```python
from build123d import *

# Parameters (mm, degrees)
F0_W      = 270
F0_H      = 280
F1_DEPTH  = 3
F2_R      = 2.25
F3_DEPTH  = 3.001
F4_R      = 2.25
F5_DEPTH  = 3.001
F7_DEPTH  = 3.001
F8_DEPTH  = 100
F9_R      = 2.25
F10_DEPTH = 3.001
F11_W     = 18
F11_H     = 20
F12_DEPTH = 3.001
F13_R     = 15


with BuildPart() as f1:
    # F0 (on Top) → F1 (new body)
    with BuildSketch(Plane.XY):
        Rectangle(F0_W, F0_H)
    extrude(amount=F1_DEPTH)

    # F2 (on face) → F3 (cut, through all)
    with BuildSketch(Plane.XY.offset(3)):
        with Locations((-16, -130)):
            Circle(F2_R)
        with Locations((-16, -90)):
            Circle(F2_R)
        with Locations((16, -130)):
            Circle(F2_R)
        with Locations((16, -90)):
            Circle(F2_R)
        with Locations((16, 118)):
            Circle(F2_R)
        with Locations((16, 78)):
            Circle(F2_R)
        with Locations((-16, 78)):
            Circle(F2_R)
        with Locations((-16, 118)):
            Circle(F2_R)
    extrude(amount=-F3_DEPTH, mode=Mode.SUBTRACT)

    # F4 (on face) → F5 (cut, through all)
    with BuildSketch(Plane.XY.offset(3)):
        with Locations((-120, 70)):
            Circle(F4_R)
        with Locations((-120, 130)):
            Circle(F4_R)
        with Locations((-88, 70)):
            Circle(F4_R)
        with Locations((-88, 130)):
            Circle(F4_R)
        with Locations((120, 130)):
            Circle(F4_R)
        with Locations((88, 130)):
            Circle(F4_R)
        with Locations((88, 70)):
            Circle(F4_R)
        with Locations((120, 70)):
            Circle(F4_R)
    extrude(amount=-F5_DEPTH, mode=Mode.SUBTRACT)

    # F6 (on face) → F7 (cut, through all)
    with BuildSketch(Plane.XY.offset(3)):
        Polygon((-135, -140), (-25, -140), (-135, 20), align=None)
        Polygon((135, 20), (25, -140), (135, -140), align=None)
    extrude(amount=-F7_DEPTH, mode=Mode.SUBTRACT)

    # F8 (add): a face of the model
    f8_faces = [f1.faces().sort_by_distance(p)[0] for p in [
        (0, 140, 1.5),
    ]]
    extrude(f8_faces, amount=F8_DEPTH)

    # F9 (on face) → F10 (cut, through all)
    with BuildSketch(Plane.XY.offset(3)):
        with Locations((125, 230)):
            Circle(F9_R)
        with Locations((125, 190)):
            Circle(F9_R)
        with Locations((93, 230)):
            Circle(F9_R)
        with Locations((93, 190)):
            Circle(F9_R)
        with Locations((-93, 230)):
            Circle(F9_R)
        with Locations((-93, 190)):
            Circle(F9_R)
        with Locations((-125, 190)):
            Circle(F9_R)
        with Locations((-125, 230)):
            Circle(F9_R)
    extrude(amount=-F10_DEPTH, mode=Mode.SUBTRACT)

    # F11 (on face) → F12 (cut, through all)
    with BuildSketch(Plane.XY.offset(3)):
        with Locations((-109, 217)):
            Rectangle(F11_W, F11_H)
        with Locations((109, 217)):
            Rectangle(F11_W, F11_H)
    extrude(amount=-F12_DEPTH, mode=Mode.SUBTRACT)

    # F13
    f13_edges = [f1.edges().sort_by_distance(p)[0] for p in [
        (-25, -140, 1.5),
        (25, -140, 1.5),
        (135, 20, 1.5),
        (135, 240, 1.5),
        (-135, 240, 1.5),
        (-135, 20, 1.5),
    ]]
    fillet(f13_edges, radius=F13_R)


solid = f1.part
```
Can you work these out from the model? Positions are in its coordinate system, mm. Round coordinates to 2 decimals unless told otherwise and drop trailing zeros. Loops run counter-clockwise (first coordinate to the right, second up) from the corner with the lowest first, then second, coordinate; pieces in that order, holes last. Notation, with made-up numbers: (12, -33.75) -> (39, -33.75) arc R13 ccw to (39, -19.75) -> close; hole circle Ø8 at (64, -16.5). An arc over 180 degrees is marked (long way). One line per item, written item: value. Start each with the question number.
1. If we section it at B-B, the plane x = 40.5: Write out the boundary of the cut face in (y, z).
2. If we section it at C-C, the plane y = -34: Write out the boundary of the cut face in (x, z) (3 decimals), then the cut area to 3 significant figures.
3. If I drill on probe 1 along X at (y, z) = (212.5, 1.7); probe 2 along Y at (x, z) = (16, 2.35); probe 3 along X at (y, z) = (130, 0.9), over which ranges is the centre line in solid material (lowest first)?
4. For pin 1 (3.5 mm diameter, centred on x = 120, y = 130, fed in from -Z); pin 2 (1.5 mm diameter, centred on y = -31.5, z = 1.5, fed in from +X); pin 3 (1.5 mm diameter, centred on y = 1, z = 1, fed in from +X), each with a flat end and sliding along its axis, tell me the tip position at first contact or that it passes through.
5. If we section it at A-A, the plane z = 2: Give the number of separate pieces and of enclosed holes in the cut face, then the cut area to 3 significant figures.
Calculated:
1. outline: (-117.45, 0) -> (240, 0) -> (240, 3) -> (-117.45, 3) -> close
2. outline: (-97.875, 0) -> (97.875, 0) -> (97.875, 3) -> (-97.875, 3) -> close
2. area: 587 mm²
3. probe 1: x = -135 to -118, -100 to 100, 118 to 135
3. probe 2: y = -140 to -132.25, -127.75 to -92.25, -87.75 to 75.75, 80.25 to 115.75, 120.25 to 240
3. probe 3: x = -135 to -122.25, -117.75 to -90.25, -85.75 to 85.75, 90.25 to 117.75, 122.25 to 135
4. pin 1: passes through
4. pin 2: stops at x = 100.11
4. pin 3: stops at x = 122.45
5. separate pieces: 1
5. enclosed holes: 26
5. area: 83,800 mm²
